Design review of the part built by this model. Coordinates are the model's own, in mm. A direction names the side the tool comes from. Coordinates: 2 decimals unless noted, no trailing zeros. Loops run counter-clockwise (first coordinate to the right, second up) from the corner with the lowest first, then second, coordinate; pieces in that order, holes last.
Q1. Add section B-B on y = 19.5. Give the boundary of the cut face in (x, z), and give its area (3 significant figures).
Q2. Add section A-A on z = 50. Give the boundary of the cut face in (x, y).
Q3. Draft analysis for pull direction Z (two halves, no side actions). For faces 1 (the face through (-15, 15, -71)), 2 (the face through (50, 13, -77)), state which applies: released by +Z, released by -Z, zero draft, split by the parting line, or undercut.
Q4. Machinability: for faces 3 (the face through (-48, 4, 43.84)), 4 (the face through (33, 21, -75)), 5 (the face through (48, 4, 64.16)), 6 (the face through (-32, 5, 0)), which of the approach directions +Z, -Z, +X, -X, +Y, -Y give a long, thin tool a straight path to every point of the face, cutting with its end or side? Answer none if there is none.
Q5. Add section C-C on z = -6. Give the boundary of the cut face in (x, y).
Q6. Wall thickness on probe 1 along X at (y, z) = (6, -69); probe 2 along Z at (x, y) = (18.5, 13); probe 3 along Z at (x, y) = (36, 4): over which ranges is each line inside the solid? List them lowest first.
Q7. For P1, Ø5, axis at x = -26.5, z = -32.5, coming from the +Y side; P2, Ø6.5, axis at y = 5.5, z = -54.5, coming from the -X side; P3, Ø1, axis at x = 4, y = 7.5, coming from the +Z side; P4, Ø3, axis at x = 36, z = 69, coming from the -Y side, all flat-tipped, find the tip position at first contact; note any pin that passes through.
```python
from build123d import *

# Parameters (mm, degrees)
SKETCH_1_W               = 100
SKETCH_1_H               = 150
EXTRUDE_2_DEPTH          = 8
SKETCH_3_R               = 1.75
CUT_EXTRUDE_1_DEPTH      = 91.493093659
MIRROR_2_COPY_1_SKETCH_R = 1.75
MIRROR_2_COPY_1_DEPTH    = 91.493093659
SKETCH_4_W               = 25
SKETCH_4_H               = 62
CUT_EXTRUDE_2_DEPTH      = 2
SKETCH_6_R               = 1.25
CUT_EXTRUDE_3_DEPTH      = 3
SKETCH_7_W               = 10
SKETCH_7_H               = 26
EXTRUDE_3_DEPTH          = 26
SKETCH_8_W               = 30
SKETCH_8_H               = 15
EXTRUDE_4_DEPTH          = 26
SKETCH_9_W               = 16
SKETCH_9_H               = 25
CUT_EXTRUDE_4_DEPTH      = 3
SKETCH_11_W              = 100
SKETCH_11_H              = 34
EXTRUDE_5_DEPTH          = 10
SKETCH_12_W              = 100
SKETCH_12_H              = 34
EXTRUDE_6_DEPTH          = 10
SKETCH_13_W              = 26
SKETCH_13_H              = 28
CUT_EXTRUDE_5_DEPTH      = 3
CUT_EXTRUDE_6_REACH      = 179.609
SKETCH_14_W              = 26
SKETCH_14_H              = 6
CUT_EXTRUDE_7_REACH      = 114.276
CUT_EXTRUDE_8_REACH      = 114.276
SKETCH_19_R              = 1.25
CUT_EXTRUDE_9_DEPTH      = 3
SKETCH_20_W              = 5
SKETCH_20_H              = 20.32
CUT_EXTRUDE_10_DEPTH     = 10
MIRROR_4_COPY_1_SKETCH_W = 5
MIRROR_4_COPY_1_SKETCH_H = 20.32
MIRROR_4_COPY_1_DEPTH    = 10
FILLET_1_R               = 10
FILLET_2_R               = 10
FILLET_3_R               = 20
FILLET_START             = -1
FILLET_4_DEPTH           = 36
FILLET_5_R               = 10
SKETCH_21_R              = 5
CUT_EXTRUDE_11_DEPTH     = 102.985293215


with BuildPart() as part:
    # 草图1 → 凸台-拉伸2 (new body)
    with BuildSketch(Plane(origin=(0, 0, 0), x_dir=(1, 0, 0), z_dir=(0, 1, 0))):
        Rectangle(SKETCH_1_W, SKETCH_1_H)
    extrude(amount=EXTRUDE_2_DEPTH)

    # 草图3 → 切除-拉伸1 (cut, through all)
    with BuildSketch(Plane(origin=(0, 8, 0), x_dir=(1, 0, 0), z_dir=(0, 1, 0))):
        with Locations(Location((-36, -19, 0), (0, 0, 270))):
            Circle(SKETCH_3_R)
        with Locations(Location((-36, -69, 0), (0, 0, 270))):
            Circle(SKETCH_3_R)
    cut_extrude_1 = extrude(amount=-CUT_EXTRUDE_1_DEPTH, mode=Mode.SUBTRACT)

    # 镜向1: 切除-拉伸1 across plane
    add(cut_extrude_1.mirror(Plane(origin=(0, 0, 0), x_dir=(0, 0, 1), z_dir=(1, 0, 0))), mode=Mode.SUBTRACT)

    # 镜向2: 切除-拉伸1 across plane
    add(cut_extrude_1.mirror(Plane.XY), mode=Mode.SUBTRACT)

    # 镜向2 copy 1 sketch → 镜向2 copy 1 (cut, through all)
    with BuildSketch(Plane(origin=(0, 8, 0), x_dir=(-1, 0, 0), z_dir=(0, 1, 0))):
        with Locations(Location((-36, -19, 0), (0, 0, 270))):
            Circle(MIRROR_2_COPY_1_SKETCH_R)
        with Locations(Location((-36, -69, 0), (0, 0, 270))):
            Circle(MIRROR_2_COPY_1_SKETCH_R)
    extrude(amount=-MIRROR_2_COPY_1_DEPTH, mode=Mode.SUBTRACT)

    # 草图4 → 切除-拉伸2 (cut)
    with BuildSketch(Plane(origin=(0, 8, 0), x_dir=(1, 0, 0), z_dir=(0, 1, 0))):
        Rectangle(SKETCH_4_W, SKETCH_4_H)
    extrude(amount=-CUT_EXTRUDE_2_DEPTH, mode=Mode.SUBTRACT)

    # 草图6 → 切除-拉伸3 (cut)
    with BuildSketch(Plane(origin=(0, 6, 0), x_dir=(1, 0, 0), z_dir=(0, 1, 0))):
        with Locations(Location((-10.5, 29, 0), (0, 0, 270))):
            Circle(SKETCH_6_R)
        with Locations(Location((10.5, 29, 0), (0, 0, 90))):
            Circle(SKETCH_6_R)
        with Locations(Location((10.5, -29, 0), (0, 0, 270))):
            Circle(SKETCH_6_R)
        with Locations(Location((-10.5, -29, 0), (0, 0, 90))):
            Circle(SKETCH_6_R)
    extrude(amount=-CUT_EXTRUDE_3_DEPTH, mode=Mode.SUBTRACT)

    # 草图7 → 凸台-拉伸3 (add)
    with BuildSketch(Plane(origin=(0, 8, 0), x_dir=(1, 0, 0), z_dir=(0, 1, 0))):
        with Locations((-45, 0)):
            Rectangle(SKETCH_7_W, SKETCH_7_H)
        with Locations((45, 0)):
            Rectangle(SKETCH_7_W, SKETCH_7_H)
    extrude(amount=EXTRUDE_3_DEPTH)

    # 草图8 → 凸台-拉伸4 (add)
    with BuildSketch(Plane(origin=(0, 8, 0), x_dir=(1, 0, 0), z_dir=(0, 1, 0))):
        with Locations((0, 67.5)):
            Rectangle(SKETCH_8_W, SKETCH_8_H)
        with Locations((0, -67.5)):
            Rectangle(SKETCH_8_W, SKETCH_8_H)
    extrude(amount=EXTRUDE_4_DEPTH)

    # 草图9 → 切除-拉伸4 (cut)
    with BuildSketch(Plane(origin=(0, 8, 0), x_dir=(1, 0, 0), z_dir=(0, 1, 0))):
        with Locations((-32, 0)):
            Rectangle(SKETCH_9_W, SKETCH_9_H)
        with Locations((32, 0)):
            Rectangle(SKETCH_9_W, SKETCH_9_H)
    extrude(amount=-CUT_EXTRUDE_4_DEPTH, mode=Mode.SUBTRACT)

    # 草图11 → 凸台-拉伸5 (add)
    with BuildSketch(Plane(origin=(0, 0, -75), x_dir=(-1, 0, 0), z_dir=(0, 0, -1))):
        with Locations((0, 17)):
            Rectangle(SKETCH_11_W, SKETCH_11_H)
    extrude(amount=EXTRUDE_5_DEPTH)

    # 草图12 → 凸台-拉伸6 (add)
    with BuildSketch(Plane.XY.offset(75)):
        with Locations((0, 17)):
            Rectangle(SKETCH_12_W, SKETCH_12_H)
    extrude(amount=EXTRUDE_6_DEPTH)

    # 草图13 → 切除-拉伸5 (cut)
    with BuildSketch(Plane.XY.offset(85)):
        with Locations((0, 20)):
            Rectangle(SKETCH_13_W, SKETCH_13_H)
    extrude(amount=-CUT_EXTRUDE_5_DEPTH, mode=Mode.SUBTRACT)

    # 草图14 → 切除-拉伸6 (cut, up to next)
    with BuildSketch(Plane.XY.offset(82), mode=Mode.PRIVATE) as cut_extrude_6_sk1:
        with Locations((0, 34)):
            Rectangle(SKETCH_14_W, SKETCH_14_H)
    cut_extrude_6_tool1 = extrude(cut_extrude_6_sk1.sketch, amount=-CUT_EXTRUDE_6_REACH, mode=Mode.PRIVATE) & part.part
    add(cut_extrude_6_tool1.solids().sort_by_distance((0, 34, 82))[0], mode=Mode.SUBTRACT)

    # 草图17 → 切除-拉伸7 (cut, up to next)
    with BuildSketch(Plane.ZY.offset(15), mode=Mode.PRIVATE) as cut_extrude_7_sk1:
        Polygon((75, 34), (60, 8), (60, 34), align=None)
    cut_extrude_7_tool1 = extrude(cut_extrude_7_sk1.sketch, amount=-CUT_EXTRUDE_7_REACH, mode=Mode.PRIVATE) & part.part
    add(cut_extrude_7_tool1.solids().sort_by_distance((-15, 25.333333, 65))[0], mode=Mode.SUBTRACT)

    # 草图18 → 切除-拉伸8 (cut, up to next)
    with BuildSketch(Plane.ZY.offset(15), mode=Mode.PRIVATE) as cut_extrude_8_sk1:
        Polygon((-75, 34), (-60, 8), (-60, 34), align=None)
    cut_extrude_8_tool1 = extrude(cut_extrude_8_sk1.sketch, amount=-CUT_EXTRUDE_8_REACH, mode=Mode.PRIVATE) & part.part
    add(cut_extrude_8_tool1.solids().sort_by_distance((-15, 25.333333, -65))[0], mode=Mode.SUBTRACT)

    # 草图19 → 切除-拉伸9 (cut)
    with BuildSketch(Plane.XY.offset(82)):
        with Locations((-10.6, 8.4)):
            Circle(SKETCH_19_R)
        with Locations(Location((10.6, 8.4, 0), (0, 0, 180))):
            Circle(SKETCH_19_R)
    extrude(amount=-CUT_EXTRUDE_9_DEPTH, mode=Mode.SUBTRACT)

    # 草图20 → 切除-拉伸10 (cut)
    with BuildSketch(Plane(origin=(0, 8, 0), x_dir=(1, 0, 0), z_dir=(0, 1, 0))):
        with Locations((-47.5, -54)):
            Rectangle(SKETCH_20_W, SKETCH_20_H)
    cut_extrude_10 = extrude(amount=-CUT_EXTRUDE_10_DEPTH, mode=Mode.SUBTRACT)

    # 镜向3: 切除-拉伸10 across plane
    add(cut_extrude_10.mirror(Plane.XY), mode=Mode.SUBTRACT)

    # 镜向4: 切除-拉伸10 across plane
    add(cut_extrude_10.mirror(Plane(origin=(0, 0, 0), x_dir=(0, 0, 1), z_dir=(1, 0, 0))), mode=Mode.SUBTRACT)

    # 镜向4 copy 1 sketch → 镜向4 copy 1 (cut)
    with BuildSketch(Plane(origin=(0, 8, 0), x_dir=(-1, 0, 0), z_dir=(0, 1, 0))):
        with Locations((-47.5, -54)):
            Rectangle(MIRROR_4_COPY_1_SKETCH_W, MIRROR_4_COPY_1_SKETCH_H)
    extrude(amount=-MIRROR_4_COPY_1_DEPTH, mode=Mode.SUBTRACT)

    # 圆角1
    # the kernel refuses this fillet: 10 mm, written as the material it takes off along each edge
    with BuildSketch(Plane(origin=(75, 0, 85), x_dir=(0, 0, -1), z_dir=(-1, 0, 0))) as fillet_1_piece_1:
        with BuildLine():
            CenterArc((FILLET_1_R, -FILLET_1_R), FILLET_1_R, 90, 90)
            Line((0, -FILLET_1_R), (0, 0))
            Line((0, 0), (FILLET_1_R, 0))
        make_face()
    extrude(amount=150, mode=Mode.SUBTRACT)

    # 圆角2
    fillet_2_edges = [part.edges().sort_by_distance(p)[0] for p in [
        (31.5, 34, 85),
        (-31.5, 34, 85),
    ]]
    fillet(fillet_2_edges, radius=FILLET_2_R - 0.0001)  # a hair under: the kernel refuses the full size

    # 圆角3
    # the kernel refuses this fillet: 20 mm, written as the material it takes off along each edge
    with BuildSketch(Plane(origin=(50, 74.0001, 85), x_dir=(0, 0, -1), z_dir=(0, -1, 0))) as fillet_3_piece_1:
        with BuildLine():
            CenterArc((FILLET_3_R, -FILLET_3_R), FILLET_3_R, 90, 90)
            Line((0, -FILLET_3_R), (0, 0))
            Line((0, 0), (FILLET_3_R, 0))
        make_face()
    extrude(amount=114.0001, mode=Mode.SUBTRACT)

    # 圆角4: read off the stored shape, not the designer's step
    # 圆角4 outline → 圆角4 (cut)
    with BuildSketch(Plane(origin=(0, 0, 0), x_dir=(1, 0, 0), z_dir=(0, 1, 0)).offset(FILLET_START)):
        with BuildLine():
            ThreePointArc((-30, -85), (-44.142135624, -79.142135624), (-50, -65))
            Line((-50, -65), (-50, -85))
            Line((-50, -85), (-30, -85))
        make_face()
    extrude(amount=FILLET_4_DEPTH, mode=Mode.SUBTRACT)

    # 圆角5
    fillet_5_edges = [part.edges().sort_by_distance(p)[0] for p in [
        (0, 0, -85),
        (0, 34, -85),
    ]]
    fillet(fillet_5_edges, radius=FILLET_5_R - 0.0001)  # a hair under: the kernel refuses the full size

    # 草图21 → 切除-拉伸11 (cut, through all)
    with BuildSketch(Plane(origin=(0, 8, 0), x_dir=(1, 0, 0), z_dir=(0, 1, 0))):
        with Locations(Location((0, 50, 0), (0, 0, 270))):
            Circle(SKETCH_21_R)
        with Locations(Location((0, -50, 0), (0, 0, 90))):
            Circle(SKETCH_21_R)
    extrude(amount=-CUT_EXTRUDE_11_DEPTH, mode=Mode.SUBTRACT)


solid = part.part
```
Entries:
1. outline: (-50, -85) - (50, -85) - (50, -75) - (15, -75) - (15, -66.63) - (-15, -66.63) - (-15, -75) - (-50, -75) - close; (-50, -13) - (-40, -13) - (-40, 13) - (-50, 13) - close; (-47.32, 75) - (-15, 75) - (-15, 66.63) - (15, 66.63) - (15, 75) - (47.32, 75) arc R20 ccw to (30, 85) - (13, 85) - (13, 82) - (-13, 82) - (-13, 85) - (-30, 85) arc R20 ccw to start; (40, -13) - (50, -13) - (50, 13) - (40, 13) - close
1. area: 2,790 mm2
2. outline: (-45, 0) - (-5, 0) - (-5, 8) - (-45, 8) - close; (5, 0) - (45, 0) - (45, 8) - (5, 8) - close
3. face 1: undercut
3. face 2: zero draft
4. face 3: -X, +Y, -Y
4. face 4: +X, +Y
4. face 5: +X, +Y, -Y
4. face 6: +Y
5. outline: (-50, 0) - (50, 0) - (50, 34) - (40, 34) - (40, 5) - (24, 5) - (24, 8) - (12.5, 8) - (12.5, 6) - (-12.5, 6) - (-12.5, 8) - (-24, 8) - (-24, 5) - (-40, 5) - (-40, 34) - (-50, 34) - close
6. probe 1: x = -50 to -37.75, -34.25 to 34.25, 37.75 to 50
6. probe 2: z = -85 to -75, 75 to 85
6. probe 3: z = -83 to -70.75, -67.25 to -20.75, -17.25 to 17.25, 20.75 to 67.25, 70.75 to 83
7. P1: stops at y = 8
7. P2: stops at x = -45
7. P3: stops at z = 82
7. P4: passes through
